Part model, mm, in its own coordinate system. A direction names the side the tool comes from. Coordinates: 2 decimals unless noted, no trailing zeros. Write each loop counter-clockwise with the first axis right and the second up, starting at its lowest first coordinate (ties: lowest second). Pieces come first, ordered by that corner, then holes. Notation, with made-up numbers: (-39.75, 22.5) -> (-14.75, 22.5) arc R22 ccw to (-14.75, 56.5) -> close; hole circle Ø4 at (6, 11.25). An arc over 180 degrees is marked (long way). One line per question, with ' | ' between items. Start each with the question number.
Item 1: Pin check, flat tips, straight feed: pin 1 (8 mm diameter, centred on y = -5, z = -13, fed in from -X); pin 2 (1.5 mm diameter, centred on y = 0, z = -3, fed in from -X); pin 3 (3 mm diameter, centred on y = 0.5, z = -5, fed in from +X). Stop position of each tip, or through.
Item 2: Saw through at C-C (x = -7.25). List the corners of the cut face in (y, z).
Item 3: Saw through at A-A (z = -5.75). List the corners of the cut face in (x, y), and give its area (3 significant figures).
Item 4: Saw through at B-B (y = 0). List the corners of the cut face in (x, z).
Item 5: Probe probe 1 along Z at (x, y) = (9.25, 0.75); probe 2 along Y at (x, z) = (-1.5, -1.25); probe 3 along X at (y, z) = (-1.75, -1.5). List the from-to ranges inside material, lowest first. Write a range as [from, to].
Item 6: 3-axis set-ups, long thin cutter, end or side, ignore diameter. For faces 4 (the flat face through (-4.191, -7.396, -5.324)), 5 (the flat face through (4.309, -7.327, -5.324)), 6 (the flat face through (4.9, 7.4, -10.5)), 7 (the flat face through (4.191, 7.396, -5.324)), 8 (the flat face through (-4.309, 7.327, -5.324)): which of +Z, -Z, +X, -X, +Y, -Y reach the whole face in a straight line?
Item 7: Two-plate mould, pull along X, no slides. Class faces 1 (the cylindrical face through (0.9, -4.05, -7.59)), 2 (the flat face through (-2, -5, -15)), 3 (the flat face through (8.5, 0, -5)): pulls with the +X half, pulls with the -X half, needs draft (parallel to the pull), parting line crosses it, or undercut.
Item 8: Saw through at D-D (y = 8.5). List the corners of the cut face in (x, z).
from build123d import *

# Parameters (mm, degrees)
SKETCH_1_W          = 11
SKETCH_1_H          = 4.5
EXTRUDE_1_DEPTH     = 10.5
HOLE_WIZARD_1_D     = 8.3
HOLE_WIZARD_1_DEPTH = 15
CHAMFER_1_SIZE      = 0.812


with BuildPart() as part:
    # 草圖1 → 旋轉1 (revolve)
    with BuildSketch(Plane(origin=(0, 0, 0), x_dir=(1, 0, 0), z_dir=(0, 1, 0))):
        with Locations((5.5, 12.75)):
            Rectangle(SKETCH_1_W, SKETCH_1_H)
    revolve(axis=Axis((0, 0, -15), (0, 0, 1)))

    # 草圖2 → 填料-伸長1 (add)
    with BuildSketch(Plane.XY.offset(-10.5)):
        Polygon((-8.5, -4.907477288), (-8.5, 4.907477288), (0, 9.814954576), (8.5, 4.907477288), (8.5, -4.907477288), (0, -9.814954576), align=None)
    extrude(amount=EXTRUDE_1_DEPTH)

    # 鑽孔1
    with Locations(Plane.XY):
        with Locations((0, 0)):
            Hole(HOLE_WIZARD_1_D / 2, depth=HOLE_WIZARD_1_DEPTH)

    # 導角1
    chamfer_1_edges = [part.edges().sort_by_distance(p)[0] for p in [
        (4.15, 0, 0),
        (4.15, 0, -15),
    ]]
    chamfer(chamfer_1_edges, length=CHAMFER_1_SIZE)


solid = part.part
From the geometry:
1) pin 1: x = -10.95 | pin 2: x = -8.5 | pin 3: x = 8.5
2) outline: (-8.27, -15) -> (8.27, -15) -> (8.27, -10.5) -> (5.63, -10.5) -> (5.63, 0) -> (-5.63, 0) -> (-5.63, -10.5) -> (-8.27, -10.5) -> close
3) outline: (-8.5, -4.91) -> (0, -9.81) -> (8.5, -4.91) -> (8.5, 4.91) -> (0, 9.81) -> (-8.5, 4.91) -> close; hole circle Ø8.3 at (0, 0) | area: 196 mm2
4) outline: (-11, -15) -> (-4.96, -15) -> (-4.15, -14.19) -> (-4.15, -0.81) -> (-4.96, 0) -> (-8.5, 0) -> (-8.5, -10.5) -> (-11, -10.5) -> close; (4.15, -14.19) -> (4.96, -15) -> (11, -15) -> (11, -10.5) -> (8.5, -10.5) -> (8.5, 0) -> (4.96, 0) -> (4.15, -0.81) -> close
5) probe 1: [-15, -10.5] | probe 2: [-8.95, -3.87], [3.87, 8.95] | probe 3: [-8.5, -3.76], [3.76, 8.5]
6) face 4: +Z, -X, -Y | face 5: +Z, +X, -Y | face 6: +Z | face 7: +Z, +X, +Y | face 8: +Z, -X, +Y
7) face 1: undercut | face 2: needs draft | face 3: pulls with the +X half
8) outline: (-6.98, -15) -> (6.98, -15) -> (6.98, -10.5) -> (2.28, -10.5) -> (2.28, 0) -> (-2.28, 0) -> (-2.28, -10.5) -> (-6.98, -10.5) -> close
